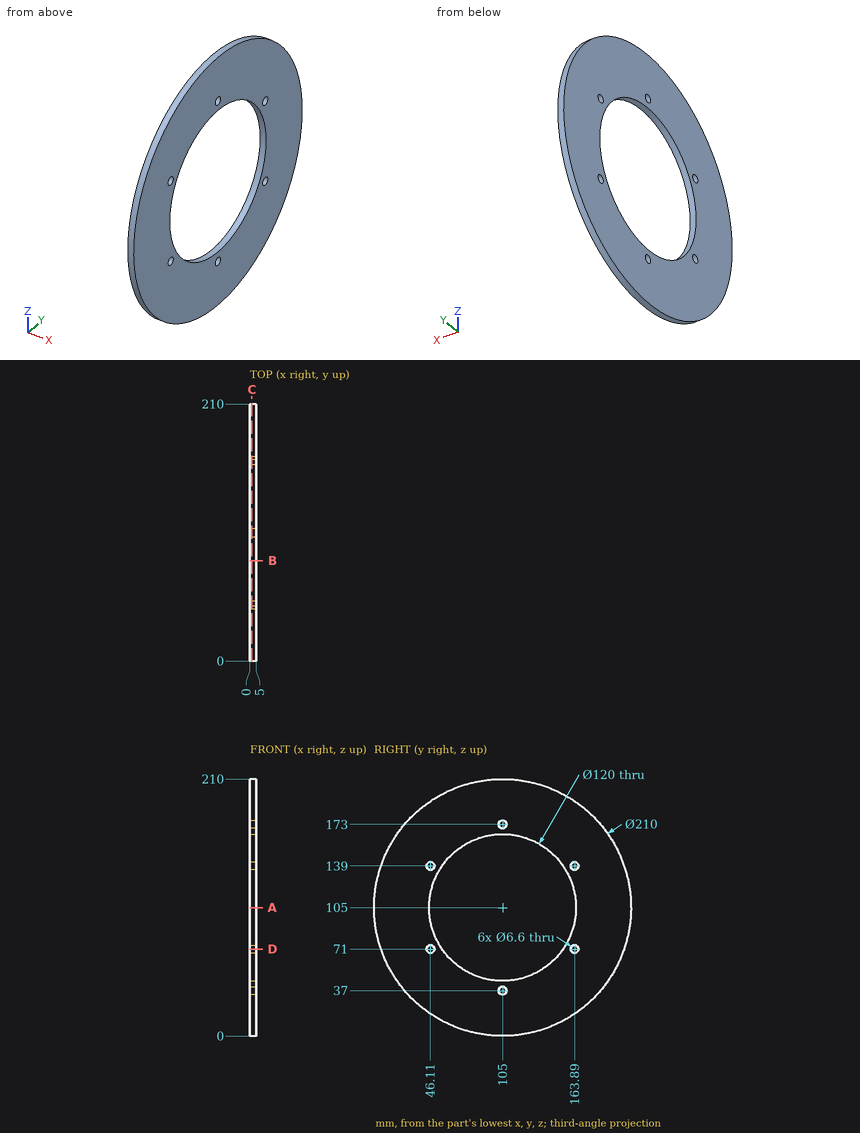
Job drawing, mm, ordinate dimensions from the low corner. One solid piece. Coordinates: 2 decimals unless noted, no trailing zeros. Write each loop counter-clockwise with the first axis right and the second up, starting at its lowest first coordinate (ties: lowest second). Pieces come first, ordered by that corner, then holes. Notation, with made-up numbers: M 13.5,-31 L 70.5,-31 A25 cw 70.5,-8 Z; hole C 50,36.25 d2. An arc over 180 degrees is marked long. Answer as a JSON object with one key per item and string values. Group by question number.
1) Pin check, flat tips, straight feed: pin 1 Ø1.5 at (x, y) = (4, 72) entering from +Z (1 decimal); pin 2 Ø6 at (y, z) = (139, 60) entering from +X. Stop position of each tip, or through.
2) Saw through at A-A (z = 105). Write the cut outline in (x, y), plus the area to 3 significant figures.
3) Saw through at B-B (y = 82). Write the cut outline in (x, z), plus the area to 3 significant figures.
4) Saw through at D-D (z = 71). Write the cut outline in (x, y).
5) Wall check: line 1 (Y direction, x = 1.4, z = 139); line 2 (Z direction, x = 2.95, y = 166) (1 decimal); line 3 (Y direction, x = 3.3, z = 105). Give the ranges that are in metal, low to high. Write a range as from..to.
6) Saw through at C-C (x = 1.65). Write the cut outline in (y, z).
Values follow:
{
 "1": {"pin 1": "stops at z = 204.9", "pin 2": "passes through"},
 "2": {"outline": "M 0,0 L 5,0 L 5,45 L 0,45 Z; M 0,165 L 5,165 L 5,210 L 0,210 Z", "area": "450 mm2"},
 "3": {"outline": "M 0,2.55 L 5,2.55 L 5,49.58 L 0,49.58 Z; M 0,160.42 L 5,160.42 L 5,207.45 L 0,207.45 Z", "area": "470 mm2"},
 "4": {"outline": "M 0,5.66 L 5,5.66 L 5,42.81 L 0,42.81 Z; M 0,49.41 L 5,49.41 L 5,55.56 L 0,55.56 Z; M 0,154.44 L 5,154.44 L 5,160.59 L 0,160.59 Z; M 0,167.19 L 5,167.19 L 5,204.34 L 0,204.34 Z"},
 "5": {"line 1": "y = 5.66..42.81, 49.41..55.56, 154.44..160.59, 167.19..204.34", "line 2": "z = 19.5..68.5, 73.5..136.5, 141.5..190.5", "line 3": "y = 0..45, 165..210"},
 "6": {"outline": "C 105,105 d210; hole C 46.11,71 d6.6; hole C 46.11,139 d6.6; hole C 105,105 d120; hole C 105,37 d6.6; hole C 105,173 d6.6; hole C 163.89,71 d6.6; hole C 163.89,139 d6.6"}
}
